Answer from the drawing. Dimensions are ordinates in mm from the lowest x, y and z of the part. Coordinates: 2 decimals unless noted, no trailing zeros. Write each loop counter-clockwise with the first axis right and the second up, starting at its lowest first coordinate (ties: lowest second). Pieces come first, ordered by that corner, then holes. Notation, with made-up numbers: (16, 34.5) -> (27, 34.5) arc R17 ccw to (27, 46.5) -> close; hole circle Ø8 at (11.25, -6.75). An arc over 180 degrees is marked (long way). Return JSON: item names as keys, results as strings.
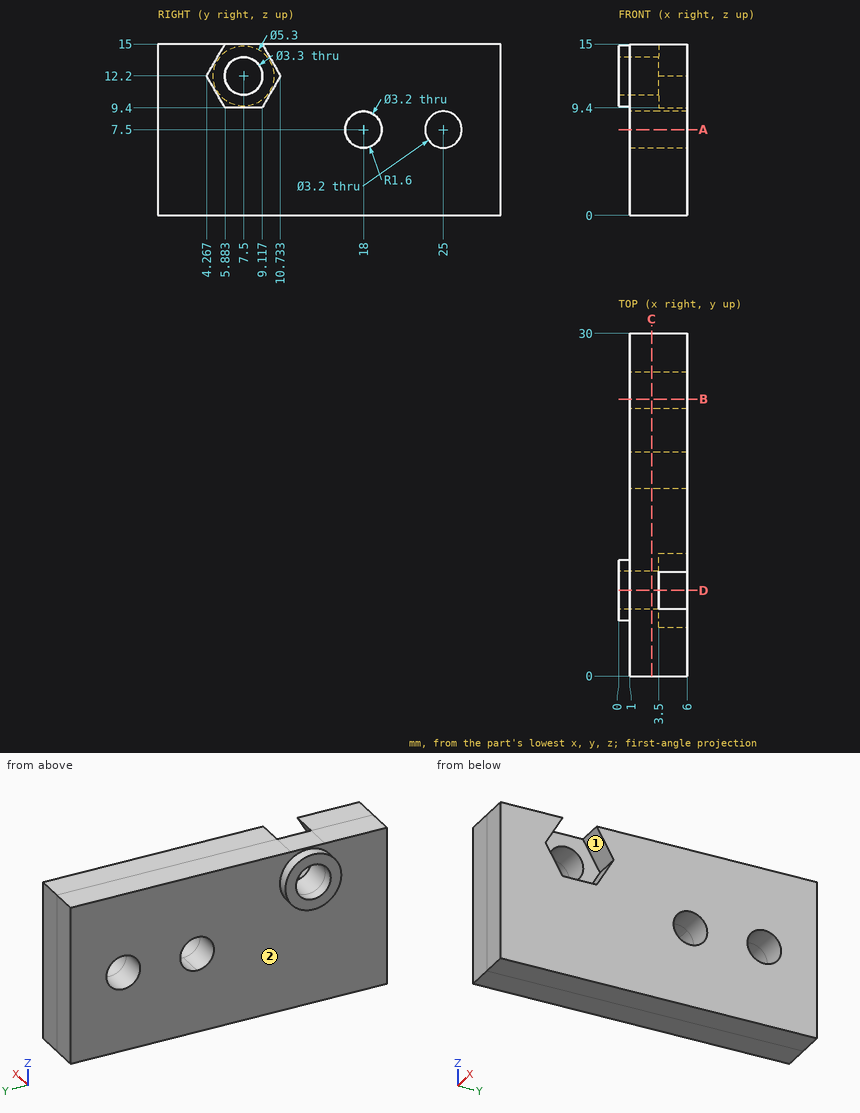
1. The part is cut by section A-A (z = 7.5). Determine the outline of the cut face in (x, y).
Taken from the geometry:
{"outline": "(1, 0) -> (6, 0) -> (6, 16.4) -> (1, 16.4) -> close; (1, 19.6) -> (6, 19.6) -> (6, 23.4) -> (1, 23.4) -> close; (1, 26.6) -> (6, 26.6) -> (6, 30) -> (1, 30) -> close"}
2. The part is cut by section C-C (x = 2.9). Determine the outline of the cut face in (y, z).
Taken from the geometry:
{"outline": "(0, 0) -> (30, 0) -> (30, 15) -> (0, 15) -> close; hole circle Ø3.3 at (7.5, 12.2); hole circle Ø3.2 at (18, 7.5); hole circle Ø3.2 at (25, 7.5)"}
3. Consider L1, parallel to Y at x = 4.2, z = 7.5; L2, parallel to Z at x = 1.25, y = 26; L3, parallel to Y at x = 2.7, z = 12.2. Determine where each line is inside the solid, lowest interval first.
Taken from the geometry:
{"L1": "y = 0 to 16.4, 19.6 to 23.4, 26.6 to 30", "L2": "z = 0 to 6.25, 8.75 to 15", "L3": "y = 0 to 5.85, 9.15 to 30"}
4. For a pull along Z with two mould halves and no side action, classify the marked faces 1 and 2 as +Z half, -Z half, draft (parallel to the pull), parting line (faces both ways), or undercut.
Taken from the geometry:
{"face 1": "undercut", "face 2": "draft"}
5. The part is cut by section D-D (y = 7.5). Determine the outline of the cut face in (x, z).
Taken from the geometry:
{"outline": "(0, 9.55) -> (1, 9.55) -> (1, 0) -> (6, 0) -> (6, 9.4) -> (3.5, 9.4) -> (3.5, 10.55) -> (0, 10.55) -> close; (0, 13.85) -> (3.5, 13.85) -> (3.5, 15) -> (1, 15) -> (1, 14.85) -> (0, 14.85) -> close"}
6. The part is cut by section B-B (y = 24.25). Determine the outline of the cut face in (x, z).
Taken from the geometry:
{"outline": "(1, 0) -> (6, 0) -> (6, 6.09) -> (1, 6.09) -> close; (1, 8.91) -> (6, 8.91) -> (6, 15) -> (1, 15) -> close"}
7. Flat-ended cylindrical pins translate along their axes: pin 1 Ø0.8 at (x, y) = (4.5, 8) entering from +Z; pin 2 Ø4 at (y, z) = (12, 7) entering from -X. Find the tip coordinate at first contact, or state that the pin passes through.
Taken from the geometry:
{"pin 1": "stops at z = 9.4", "pin 2": "stops at x = 1"}
